Source: three-view drawing plus pictorial views. Frame: mm from the lowest corner of the part. Coordinates: 2 decimals unless noted, no trailing zeros. Order: outer loops, then holes, each group sorted by start corner. A loop starts at its lowest first (then second) coordinate and runs counter-clockwise, first axis right, second up. Notation, with made-up numbers: M 59,80.25 L 69,80.25 A23 cw 69,113.25 Z; hole C 37.5,19 d10. An arc over 180 degrees is marked long. Write item = value, one per line. Start each with the question number.
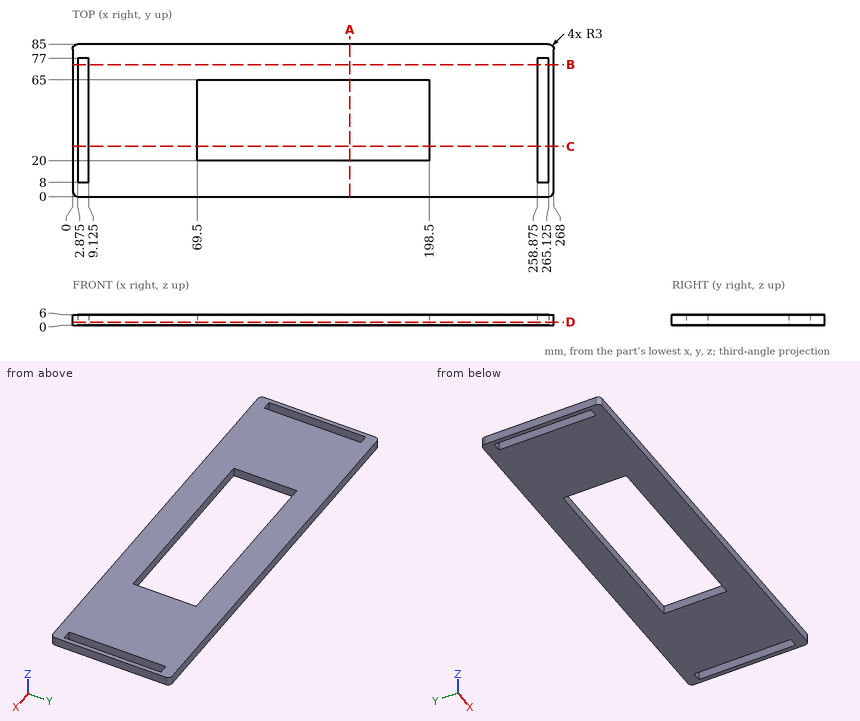
Item 1: Section query B-B on y = 73.5. Output: boundary loops of the cut face in (x, z) (3 decimals), and give its area (3 significant figures).
Item 2: Section query A-A on x = 154.5. Output: boundary loops of the cut face in (y, z).
Item 3: Material intervals for probe 1 along X at (y, z) = (73, 5.3) (3 decimals); probe 2 along X at (y, z) = (21, 1.45) (3 decimals); probe 3 along Y at (x, z) = (153.5, 0.6), sorted ascending. Write a range as [from, to].
Item 4: Section query C-C on y = 28. Output: boundary loops of the cut face in (x, z) (3 decimals).
Item 5: Section query D-D on z = 1.8. Output: boundary loops of the cut face in (x, y) (3 decimals).
Ans:
q1.outline = M 0,0 L 2.875,0 L 2.875,6 L 0,6 Z; M 9.125,0 L 258.875,0 L 258.875,6 L 9.125,6 Z; M 265.125,0 L 268,0 L 268,6 L 265.125,6 Z
q1.area = 1,530 mm^2
q2.outline = M 0,0 L 20,0 L 20,6 L 0,6 Z; M 65,0 L 85,0 L 85,6 L 65,6 Z
q3.probe_1 = [0, 2.875], [9.125, 258.875], [265.125, 268]
q3.probe_2 = [0, 2.875], [9.125, 69.5], [198.5, 258.875], [265.125, 268]
q3.probe_3 = [0, 20], [65, 85]
q4.outline = M 0,0 L 2.875,0 L 2.875,6 L 0,6 Z; M 9.125,0 L 69.5,0 L 69.5,6 L 9.125,6 Z; M 198.5,0 L 258.875,0 L 258.875,6 L 198.5,6 Z; M 265.125,0 L 268,0 L 268,6 L 265.125,6 Z
q5.outline = M 0,3 A3 ccw 3,0 L 265,0 A3 ccw 268,3 L 268,82 A3 ccw 265,85 L 3,85 A3 ccw 0,82 Z; hole M 2.875,8 L 9.125,8 L 9.125,77 L 2.875,77 Z; hole M 69.5,20 L 198.5,20 L 198.5,65 L 69.5,65 Z; hole M 258.875,8 L 265.125,8 L 265.125,77 L 258.875,77 Z
